```python
from build123d import *

# Parameters (mm, degrees)
F1_DEPTH = 1.27
F3_R     = 0.508
F2_R     = 0.508
F4_DEPTH = 25.4


with BuildPart() as f1:
    # F0 (on Front) → F1 (new body, symmetric)
    with BuildSketch(Plane.XZ):
        with BuildLine():
            ThreePointArc((-3.592195, -2.4189042089), (-4.1419609714, -1.2645638781), (-4.3307, 0))
            Line((-4.3307, 0), (-5.497195, 0))
            Line((-5.497195, 0), (-5.497195, -2.441702))
            Line((-5.497195, -2.441702), (-3.592195, -2.441702))
            Line((-3.592195, -2.441702), (-3.592195, -2.4189042089))
        make_face()
        with BuildLine():
            Line((5.497195, 0), (4.3307, 0))
            ThreePointArc((4.3307, 0), (4.1419609714, -1.2645638781), (3.592195, -2.4189042089))
            Line((3.592195, -2.4189042089), (3.592195, -2.441702))
            Line((3.592195, -2.441702), (5.497195, -2.441702))
            Line((5.497195, -2.441702), (5.497195, 0))
        make_face()
        with BuildLine():
            Line((-3.592195, 0), (-4.3307, 0))
            ThreePointArc((-4.3307, 0), (-4.1419609714, -1.2645638781), (-3.592195, -2.4189042089))
            Line((-3.592195, -2.4189042089), (-3.592195, 0))
        make_face()
        with BuildLine():
            ThreePointArc((3.592195, -2.4189042089), (4.1419609714, -1.2645638781), (4.3307, 0))
            Line((4.3307, 0), (3.592195, 0))
            Line((3.592195, 0), (3.592195, -2.4189042089))
        make_face()
        with BuildLine():
            ThreePointArc((-3.592195, -2.4189042089), (0, -4.3307), (3.592195, -2.4189042089))
            Line((3.592195, -2.4189042089), (3.592195, 0))
            Line((3.592195, 0), (2.7051, 0))
            ThreePointArc((2.7051, 0), (0, -2.7051), (-2.7051, 0))
            Line((-2.7051, 0), (-3.592195, 0))
            Line((-3.592195, 0), (-3.592195, -2.4189042089))
        make_face()
    extrude(amount=F1_DEPTH, both=True)

    # F3 (on face) + F2 (on face) → F4 (cut)
    with BuildSketch(Plane(origin=(0, 0, -2.441702), x_dir=(1, 0, 0), z_dir=(0, 0, -1))):
        with Locations((4.544695, 0)):
            Circle(F3_R)
    with BuildSketch(Plane(origin=(0, 0, -2.441702), x_dir=(1, 0, 0), z_dir=(0, 0, -1))):
        with Locations((-4.544695, 0)):
            Circle(F2_R)
    extrude(amount=-F4_DEPTH, mode=Mode.SUBTRACT)


solid = f1.part
```
Check sheet for the modelled part. Datum: model origin and axes. Units: mm. A direction names the side the tool comes from. Round coordinates to 2 decimals unless told otherwise and drop trailing zeros. Order: outer loops, then holes, each group sorted by start corner. A loop starts at its lowest first (then second) coordinate and runs counter-clockwise, first axis right, second up.
1) Section check A-A (y = 0). Give the number of separate pieces and of enclosed holes in the cut face, and give its area (3 significant figures).
2) Section check B-B (z = -2.1). Record the boundary of the cut face in (x, y), and give its area (3 significant figures).
3) Section check C-C (x = -4.25). Record the boundary of the cut face in (y, z), and give its area (3 significant figures).
4) Scan lines: line 1 (X direction, y = 0.1, z = -1); line 2 (X direction, y = 0, z = -1.7); line 3 (X direction, y = -0.9, z = -0.3). Record each from-to range of solid material in increasing order.
5) Section check D-D (z = -2.55). Record the boundary of the cut face in (x, y), and give its area (3 significant figures).
6) Mould release check, pull along Y, two halves, no side actions. Record for faces 1 (the flat face through (0, -1.27, -3)), 2 (the cylindrical face through (4.037, -0.022, -1.238)), 3 (the flat face through (0, 1.27, -3)), 4 (the flat face through (-3.8, 0, 0)): +Y half, -Y half, draft (parallel to the pull), parting line (faces both ways), or undercut.
7) Tool access check on faces 5 (the flat face through (5, -1, -2.442)), 6 (the flat face through (-5, -1, -2.442)), 7 (the flat face through (-5.497, 0, -1)). Record the directions out of +Z, -Z, +X, -X, +Y, -Y that give a thin tool (end or side, any length) a straight path to the whole face; none if there is none.
8) Go/stop test with flat-tipped pins: pin 1 Ø0.6 at (x, y) = (5, -0.5) entering from -Z; pin 2 Ø1.5 at (x, y) = (-4, 0) entering from -Z; pin 3 Ø1 at (x, y) = (-2.5, -0.5) entering from +Z; pin 4 Ø1.5 at (x, y) = (2.5, -1) entering from -Z. Record where each tip stops, or that it passes through.
Result:
1. separate pieces: 3
1. enclosed holes: 0
1. area: 19.9 mm2
2. outline: (-5.5, -1.27) - (-1.71, -1.27) - (-1.71, 1.27) - (-5.5, 1.27) - close; (1.71, -1.27) - (5.5, -1.27) - (5.5, 1.27) - (1.71, 1.27) - close; hole circle Ø1.02 at (-4.54, 0); hole circle Ø1.02 at (4.54, 0)
2. area: 17.6 mm2
3. outline: (-1.27, -2.44) - (-0.41, -2.44) - (-0.41, 0) - (-1.27, 0) - close; (0.41, -2.44) - (1.27, -2.44) - (1.27, 0) - (0.41, 0) - close
3. area: 4.18 mm2
4. line 1: x = -5.5 to -5.04, -4.05 to -2.51, 2.51 to 4.05, 5.04 to 5.5
4. line 2: x = -5.5 to -5.05, -4.04 to -2.1, 2.1 to 4.04, 5.05 to 5.5
4. line 3: x = -5.5 to -2.69, 2.69 to 5.5
5. outline: (-3.5, -1.27) - (-0.9, -1.27) - (-0.9, 1.27) - (-3.5, 1.27) - close; (0.9, -1.27) - (3.5, -1.27) - (3.5, 1.27) - (0.9, 1.27) - close
5. area: 13.2 mm2
6. face 1: -Y half
6. face 2: undercut
6. face 3: +Y half
6. face 4: draft
7. face 5: -Z, +X, +Y, -Y
7. face 6: -Z, -X, +Y, -Y
7. face 7: +Z, -Z, -X, +Y, -Y
8. pin 1: stops at z = -2.44
8. pin 2: stops at z = -2.86
8. pin 3: stops at z = 0
8. pin 4: stops at z = -3.96
